Build history of the part. All positions in model axes, mm. Face numbers are marked on the shaded views. A direction names the side the tool comes from. Give positions to 0.01 mm unless a question says otherwise; leave off trailing zeros. Write each loop counter-clockwise with the first axis right and the second up, starting at its lowest first coordinate (ties: lowest second). Pieces come first, ordered by that corner, then holes.
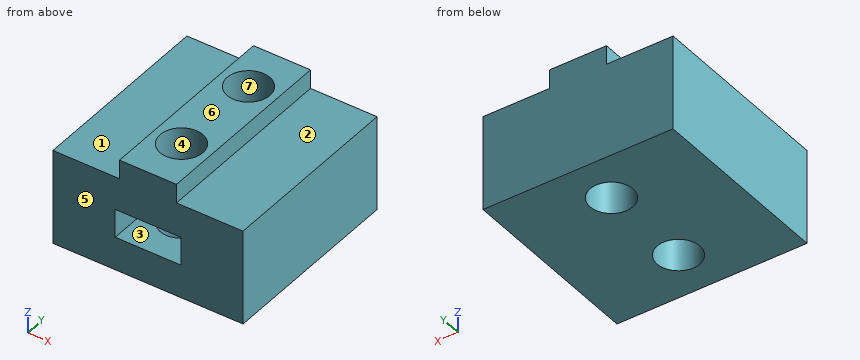
from build123d import *

# Parameters (mm, degrees)
SKETCH_W     = 20
SKETCH_H     = 20
SKETCH_R     = 2.25
PAD_DEPTH    = 10
SKETCH001_W  = 6
SKETCH001_H  = 20
SKETCH001_R  = 2.25
PAD001_DEPTH = 2
SKETCH002_W  = 6.9
SKETCH002_H  = 3
POCKET_DEPTH = 10


with BuildPart() as part:
    # Sketch → Pad (new body)
    with BuildSketch(Plane.XY):
        Rectangle(SKETCH_W, SKETCH_H)
        with Locations((0, 5)):
            Circle(SKETCH_R, mode=Mode.SUBTRACT)
        with Locations((0, -5)):
            Circle(SKETCH_R, mode=Mode.SUBTRACT)
    extrude(amount=PAD_DEPTH)

    # Sketch001 → Pad001 (new body)
    with BuildSketch(Plane.XY.offset(10)):
        Rectangle(SKETCH001_W, SKETCH001_H)
        with Locations((0, 5)):
            Circle(SKETCH001_R, mode=Mode.SUBTRACT)
        with Locations((0, -5)):
            Circle(SKETCH001_R, mode=Mode.SUBTRACT)
    extrude(amount=PAD001_DEPTH)

    # Sketch002 → Pocket (cut)
    with BuildSketch(Plane.XZ.offset(10)):
        with Locations((0, 5)):
            Rectangle(SKETCH002_W, SKETCH002_H)
    extrude(amount=-POCKET_DEPTH, mode=Mode.SUBTRACT)


solid = part.part
(1) Saw through at A-A, the plane y = -5. List the corners of the cut face in (x, z), plus the area to 3 significant figures.
(2) Drop flat-ended pins along their axis: pin 1 (0.6 mm diameter, centred on y = 1, z = 11, fed in from -X); pin 2 (1.5 mm diameter, centred on x = 1.5, z = 5, fed in from -Y); pin 3 (3.5 mm diameter, centred on x = 5.5, y = -0.5, fed in from +Z). Give the stop position or say it passes through.
(3) Saw through at C-C, the plane z = 5.5. List the corners of the cut face in (x, y), plus the area to 3 significant figures.
(4) Saw through at D-D, the plane y = 5. List the corners of the cut face in (x, z).
(5) Probe line 1 (Y direction, x = 0, z = 3.25); line 2 (X direction, y = -4.5, z = 5.25); line 3 (X direction, y = -5, z = 8.3). List the from-to ranges inside material, lowest first.
(6) Mould opens along Y. For the marked faces 4, 5, 6 and 7 say: +Y half, -Y half, draft (parallel to the pull), parting line (faces both ways), or undercut.
(7) Saw through at B-B, the plane x = 0. List the corners of the cut face in (y, z), plus the area to 4 significant figures.
(8) 3-axis set-ups, long thin cutter, end or side, ignore diameter. For the marked faces 1, 2 and 3: which of +Z, -Z, +X, -X, +Y, -Y reach the whole face in a straight line?
Computed values:
1. outline: (-10, 0) - (-2.25, 0) - (-2.25, 3.5) - (-3.45, 3.5) - (-3.45, 6.5) - (-2.25, 6.5) - (-2.25, 12) - (-3, 12) - (-3, 10) - (-10, 10) - close; (2.25, 0) - (10, 0) - (10, 10) - (3, 10) - (3, 12) - (2.25, 12) - (2.25, 6.5) - (3.45, 6.5) - (3.45, 3.5) - (2.25, 3.5) - close
1. area: 151 mm2
2. pin 1: stops at x = -3
2. pin 2: stops at y = 0
2. pin 3: stops at z = 10
3. outline: (-10, -10) - (-3.45, -10) - (-3.45, 0) - (3.45, 0) - (3.45, -10) - (10, -10) - (10, 10) - (-10, 10) - close; hole circle Ø4.5 at (0, 5)
3. area: 315 mm2
4. outline: (-10, 0) - (-2.25, 0) - (-2.25, 12) - (-3, 12) - (-3, 10) - (-10, 10) - close; (2.25, 0) - (10, 0) - (10, 10) - (3, 10) - (3, 12) - (2.25, 12) - close
5. line 1: y = -10 to -7.25, -2.75 to 2.75, 7.25 to 10
5. line 2: x = -10 to -3.45, 3.45 to 10
5. line 3: x = -10 to -2.25, 2.25 to 10
6. face 4: undercut
6. face 5: -Y half
6. face 6: draft
6. face 7: undercut
7. outline: (-10, 0) - (-7.25, 0) - (-7.25, 3.5) - (-10, 3.5) - close; (-10, 6.5) - (-7.25, 6.5) - (-7.25, 12) - (-10, 12) - close; (-2.75, 0) - (2.75, 0) - (2.75, 12) - (-2.75, 12) - (-2.75, 6.5) - (0, 6.5) - (0, 3.5) - (-2.75, 3.5) - close; (7.25, 0) - (10, 0) - (10, 12) - (7.25, 12) - close
7. area: 115.5 mm2
8. face 1: +Z, -X, +Y, -Y
8. face 2: +Z, +X, +Y, -Y
8. face 3: -Y
